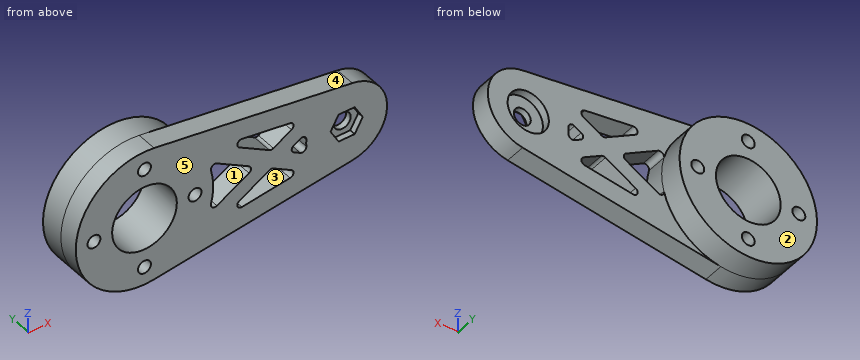
from build123d import *

# Parameters (mm, degrees)
SKETCH_1_R          = 1.6
SKETCH_1_R_2        = 8
SKETCH_1_R_3        = 5.1
EXTRUDE_1_DEPTH     = 5
SKETCH_1_3_R        = 5.1
SKETCH_1_3_R_2      = 2.1
EXTRUDE_2_DEPTH     = 3
FILLET_1_R          = 1
FILLET_2_R          = 1
FILLET_3_R          = 1
FILLET_4_R          = 1
CUT_EXTRUDE_1_DEPTH = 1.5
SKETCH_3_R          = 17
SKETCH_3_R_2        = 8
SKETCH_3_R_3        = 1.6
EXTRUDE_4_DEPTH     = 6


with BuildPart() as part:
    # Sketch 1 → Extrude 1 (new body)
    with BuildSketch(Plane(origin=(0, 0, 0), x_dir=(1, 0, 0), z_dir=(0, 1, 0))):
        with BuildLine():
            Line((2.38, -16.832575561), (51.4, -9.901515036))
            ThreePointArc((51.4, -9.901515036), (60, 0), (51.4, 9.901515036))
            Line((51.4, 9.901515036), (2.38, 16.832575561))
            ThreePointArc((2.38, 16.832575561), (-17, 0), (2.38, -16.832575561))
        make_face()
        with Locations(Location((-12.5, 0, 0), (0, 0, 270))):
            Circle(SKETCH_1_R, mode=Mode.SUBTRACT)
        with Locations(Location((0, 12.5, 0), (0, 0, 270))):
            Circle(SKETCH_1_R, mode=Mode.SUBTRACT)
        with Locations(Location((12.5, 0, 0), (0, 0, 270))):
            Circle(SKETCH_1_R, mode=Mode.SUBTRACT)
        with Locations(Location((0, -12.5, 0), (0, 0, 270))):
            Circle(SKETCH_1_R, mode=Mode.SUBTRACT)
        with Locations(Location((0, 0, 0), (0, 0, 270))):
            Circle(SKETCH_1_R_2, mode=Mode.SUBTRACT)
        with Locations(Location((50, 0, 0), (0, 0, 270))):
            Circle(SKETCH_1_R_3, mode=Mode.SUBTRACT)
        Polygon((18.93798634, 9.441668148), (38.90018853, 6.619162403), (31.379588649, 2.305623307), align=None, mode=Mode.SUBTRACT)
        Polygon((18.93798634, -9.441668148), (38.90018853, -6.619162403), (31.379588649, -2.305623307), align=None, mode=Mode.SUBTRACT)
        with BuildLine():
            Line((15.606195444, 6.741414077), (27.359764097, 0))
            Line((27.359764097, 0), (15.606195444, -6.741414077))
            ThreePointArc((15.606195444, -6.741414077), (17, 0), (15.606195444, 6.741414077))
        make_face(mode=Mode.SUBTRACT)
        with BuildLine():
            Line((35.399413201, 0), (40.424329865, -2.882107123))
            ThreePointArc((40.424329865, -2.882107123), (40, 0), (40.424329865, 2.882107123))
            Line((40.424329865, 2.882107123), (35.399413201, 0))
        make_face(mode=Mode.SUBTRACT)
    extrude(amount=EXTRUDE_1_DEPTH)

    # Sketch 1_3 → Extrude 2 (add)
    with BuildSketch(Plane(origin=(0, 0, 0), x_dir=(1, 0, 0), z_dir=(0, 1, 0))):
        with Locations(Location((50, 0, 0), (0, 0, 270))):
            Circle(SKETCH_1_3_R)
        with Locations(Location((50, 0, 0), (0, 0, 270))):
            Circle(SKETCH_1_3_R_2, mode=Mode.SUBTRACT)
    extrude(amount=EXTRUDE_2_DEPTH)

    # Fillet 1
    fillet_1_edges = [part.edges().sort_by_distance(p)[0] for p in [
        (35.399413201, 2.5, 0),
        (40.424329865, 2.5, 2.882107123),
        (40.424329865, 2.5, -2.882107123),
    ]]
    fillet(fillet_1_edges, radius=FILLET_1_R)

    # Fillet 2
    fillet_2_edges = [part.edges().sort_by_distance(p)[0] for p in [
        (18.93798634, 2.5, 9.441668148),
        (38.90018853, 2.5, 6.619162403),
        (31.379588649, 2.5, 2.305623307),
    ]]
    fillet(fillet_2_edges, radius=FILLET_2_R)

    # Fillet 3
    fillet_3_edges = [part.edges().sort_by_distance(p)[0] for p in [
        (38.90018853, 2.5, -6.619162403),
        (18.93798634, 2.5, -9.441668148),
        (31.379588649, 2.5, -2.305623307),
    ]]
    fillet(fillet_3_edges, radius=FILLET_3_R)

    # Fillet 4
    fillet_4_edges = [part.edges().sort_by_distance(p)[0] for p in [
        (27.359764097, 2.5, 0),
        (15.606195444, 2.5, -6.741414077),
        (15.606195444, 2.5, 6.741414077),
    ]]
    fillet(fillet_4_edges, radius=FILLET_4_R)

    # Sketch 2 → Cut-Extrude 1 (cut)
    with BuildSketch(Plane.XZ):
        Polygon((53.983716857, 0), (51.991858429, 3.45), (48.008141571, 3.45), (46.016283143, 0), (48.008141571, -3.45), (51.991858429, -3.45), align=None)
    extrude(amount=-CUT_EXTRUDE_1_DEPTH, mode=Mode.SUBTRACT)

    # Sketch 3 → Extrude 4 (add)
    with BuildSketch(Plane(origin=(0, 5, 0), x_dir=(1, 0, 0), z_dir=(0, 1, 0))):
        with Locations(Location((0, 0, 0), (0, 0, 81.952153753))):
            Circle(SKETCH_3_R)
        with Locations(Location((0, 0, 0), (0, 0, 270))):
            Circle(SKETCH_3_R_2, mode=Mode.SUBTRACT)
        with Locations(Location((0, -12.5, 0), (0, 0, 270))):
            Circle(SKETCH_3_R_3, mode=Mode.SUBTRACT)
        with Locations(Location((12.5, 0, 0), (0, 0, 270))):
            Circle(SKETCH_3_R_3, mode=Mode.SUBTRACT)
        with Locations(Location((0, 12.5, 0), (0, 0, 270))):
            Circle(SKETCH_3_R_3, mode=Mode.SUBTRACT)
        with Locations(Location((-12.5, 0, 0), (0, 0, 270))):
            Circle(SKETCH_3_R_3, mode=Mode.SUBTRACT)
    extrude(amount=EXTRUDE_4_DEPTH)


solid = part.part
Verification items for the finished model (mm, model axes). Face numbers are marked on the shaded views. A direction names the side the tool comes from. Coordinates: 2 decimals unless noted, no trailing zeros. Loops run counter-clockwise (first coordinate to the right, second up) from the corner with the lowest first, then second, coordinate; pieces in that order, holes last. Notation, with made-up numbers: (9, -34) -> (40, -34) arc R25 cw to (40, -6) -> close; hole circle Ø8 at (27.25, 22). An arc over 180 degrees is marked (long way). Answer as a JSON object with one key per item and string values. Group by question number.
Item 1: Sectioned sample at A-A on y = 8. Record the boundary of the cut face in (x, z), plus the area to 3 significant figures.
Item 2: Sectioned sample at B-B on z = -12.5. Record the boundary of the cut face in (x, y).
Item 3: Mould release check, pull along Z, two halves, no side actions. Record for the marked faces 3, 4 and 5: +Z half, -Z half, draft (parallel to the pull), parting line (faces both ways), or undercut.
Item 4: Sectioned sample at C-C on x = 50. Record the boundary of the cut face in (y, z), plus the area to 3 significant figures.
Item 5: Sectioned sample at D-D on x = -12.5. Record the boundary of the cut face in (y, z), plus the area to 3 significant figures.
Item 6: Scan lines: probe 1 along X at (y, z) = (5.5, 0); probe 2 along X at (y, z) = (7.5, -15); probe 3 along X at (y, z) = (5.5, 12.5). Record each from-to range of solid material in increasing order.
Item 7: Tool access check on the marked faces 1 and 2. Record the directions out of +Z, -Z, +X, -X, +Y, -Y that give a thin tool (end or side, any length) a straight path to the whole face; none if there is none.
Item 8: Depth check by flat-ended pin: pin 1 (8 mm diameter, centred on x = 48, z = -2, fed in from +Y); pin 2 (5 mm diameter, centred on x = 0, z = -12.5, fed in from +Y); pin 3 (4 mm diameter, centred on x = 50, z = 0, fed in from +Y); pin 4 (4 mm diameter, centred on y = 9, z = -11.5, fed in from +X). Enter the tip coordinate at first touch or a pass-through.
Evaluation:
{
 "1": {"outline": "circle Ø34 at (0, 0); hole circle Ø3.2 at (-12.5, 0); hole circle Ø16 at (0, 0); hole circle Ø3.2 at (0, -12.5); hole circle Ø3.2 at (0, 12.5); hole circle Ø3.2 at (12.5, 0)", "area": "675 mm²"},
 "2": {"outline": "(-11.52, 0) -> (-1.6, 0) -> (-1.6, 11) -> (-11.52, 11) -> close; (1.6, 0) -> (33.02, 0) -> (33.02, 5) -> (11.52, 5) -> (11.52, 11) -> (1.6, 11) -> close"},
 "3": {"face 3": "undercut", "face 4": "+Z half", "face 5": "draft"},
 "4": {"outline": "(0, -10.1) -> (5, -10.1) -> (5, -5.1) -> (3, -5.1) -> (3, -2.1) -> (1.5, -2.1) -> (1.5, -3.45) -> (0, -3.45) -> close; (0, 3.45) -> (1.5, 3.45) -> (1.5, 2.1) -> (3, 2.1) -> (3, 5.1) -> (5, 5.1) -> (5, 10.1) -> (0, 10.1) -> close", "area": "63.9 mm²"},
 "5": {"outline": "(0, -11.52) -> (11, -11.52) -> (11, -1.6) -> (0, -1.6) -> close; (0, 1.6) -> (11, 1.6) -> (11, 11.52) -> (0, 11.52) -> close", "area": "218 mm²"},
 "6": {"probe 1": "x = -17 to -14.1, -10.9 to -8, 8 to 10.9, 14.1 to 17", "probe 2": "x = -8 to 8", "probe 3": "x = -11.52 to -1.6, 1.6 to 11.52"},
 "7": {"face 1": "+Y, -Y", "face 2": "+Z, -Z, +X, -X, +Y"},
 "8": {"pin 1": "stops at y = 5", "pin 2": "stops at y = 11", "pin 3": "passes through", "pin 4": "stops at x = 14.1"}
}
